The drawing under review shows one solid part. Ordinate dimensions are in mm from its lowest x, y, z. Coordinates: 2 decimals unless noted, no trailing zeros. Write each loop counter-clockwise with the first axis right and the second up, starting at its lowest first coordinate (ties: lowest second). Pieces come first, ordered by that corner, then holes.
1) For line 1 (Y direction, x = 6.25, z = 3); line 2 (X direction, y = 7.25, z = 9.5); line 3 (X direction, y = 1.4, z = 15.85) (1 decimal), list the stretches that pass through material, from the lowest coordinate up.
2) Add section A-A, the plane x = 9.5. State the section outline as (y, z) points.
3) Mouldability with a two-part tool opening along Z and no side actions: class the marked faces 1, 2 and 3 as released by +Z, released by -Z, zero draft, split by the parting line, or undercut.
4) Add section C-C, the plane z = 9.5. State the section outline as (x, y) points.
5) For P1, Ø2.5, axis at x = 4, z = 6.32, coming from the -Y side; P2, Ø5, axis at x = 17, z = 14, coming from the +Y side, all flat-tipped, find the tip position at first contact; note any pin that passes through.
6) Add section B-B, the plane z = 5. State the section outline as (x, y) points (1 decimal), then the cut area to 3 significant figures.
7) Add section D-D, the plane y = 5. State the section outline as (x, z) points.
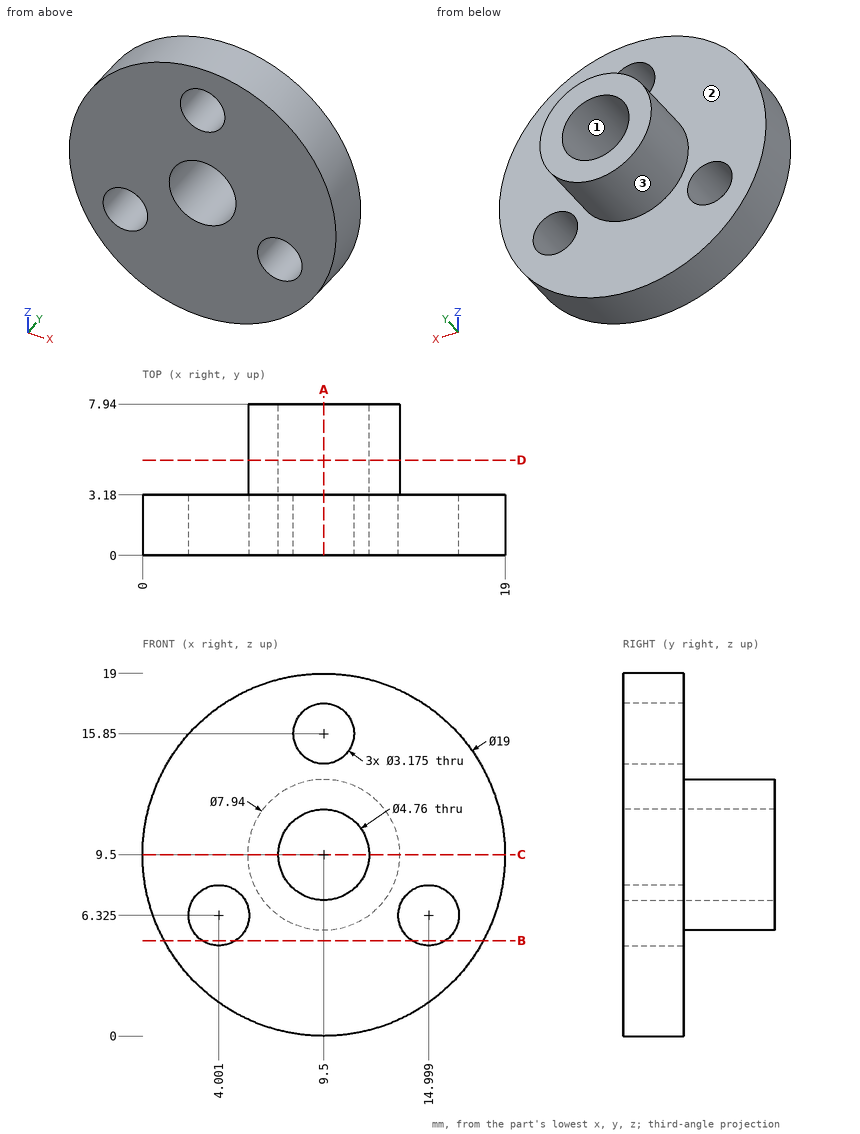
Geometry results:
1. line 1: y = 0 to 3.18
1. line 2: x = 5.53 to 7.12, 11.88 to 13.47
1. line 3: x = 2.4 to 7.9, 11.1 to 16.6
2. outline: (0, 0) - (3.18, 0) - (3.18, 5.53) - (7.94, 5.53) - (7.94, 7.12) - (0, 7.12) - close; (0, 11.88) - (7.94, 11.88) - (7.94, 13.47) - (3.18, 13.47) - (3.18, 14.26) - (0, 14.26) - close; (0, 17.44) - (3.18, 17.44) - (3.18, 19) - (0, 19) - close
3. face 1: undercut
3. face 2: zero draft
3. face 3: split by the parting line
4. outline: (0, 0) - (7.12, 0) - (7.12, 7.94) - (5.53, 7.94) - (5.53, 3.18) - (0, 3.18) - close; (11.88, 0) - (19, 0) - (19, 3.18) - (13.47, 3.18) - (13.47, 7.94) - (11.88, 7.94) - close
5. P1: passes through
5. P2: stops at y = 3.18
6. outline: (1.1, 0) - (3.1, 0) - (3.1, 3.2) - (1.1, 3.2) - close; (4.9, 0) - (14.1, 0) - (14.1, 3.2) - (4.9, 3.2) - close; (15.9, 0) - (17.9, 0) - (17.9, 3.2) - (15.9, 3.2) - close
6. area: 42.1 mm2
7. outline: circle Ø7.94 at (9.5, 9.5); hole circle Ø4.76 at (9.5, 9.5)
